Model file for the job. Use its own axes, mm. Face numbers are marked on the shaded views. A direction names the side the tool comes from. Coordinates: 2 decimals unless noted, no trailing zeros. Order: outer loops, then holes, each group sorted by start corner. A loop starts at its lowest first (then second) coordinate and runs counter-clockwise, first axis right, second up. Notation, with made-up numbers: (24, 43.25) -> (71, 43.25) arc R22 cw to (71, 59.25) -> close; hole circle Ø1 at (-1.5, 56.5). An arc over 180 degrees is marked (long way). Return JSON: item names as keys, results as strings. Group by question number.
1) Cut at B-B (y = 7.5). Write the cut outline in (x, z).
2) Which spindle directions (+Z, -Z, +X, -X, +Y, -Y) get a long thin tool onto all of the face, cutting with end or side? Do the marked faces 1, 2 and 3. Say none if no direction does.
3) Flat gauge pins, fed straight in: pin 1 (3 mm diameter, centred on x = -32, y = 3.5, fed in from +Z); pin 2 (2 mm diameter, centred on y = -9.5, z = 4, fed in from +X); pin 3 (20.5 mm diameter, centred on x = 17.5, y = 1, fed in from +Z). Where does each tip first touch, or does it go through?
4) Probe line 1 (Y direction, x = 0, z = 4); line 2 (X direction, y = -17, z = 11.5); line 3 (X direction, y = -4.5, z = 9.5). List the from-to ranges inside material, lowest first.
5) Pull direction X, two halves, no side cores. Call the marked faces 4, 5, 6 and 7: +X half, -X half, draft (parallel to the pull), parting line (faces both ways), or undercut.
6) Cut at C-C (y = 0). Write the cut outline in (x, z), and give its area (3 significant figures).
7) Cut at A-A (x = 0). Write the cut outline in (y, z), and give its area (3 significant figures).
8) Cut at D-D (x = 11). Write the cut outline in (y, z), and give its area (3 significant figures).
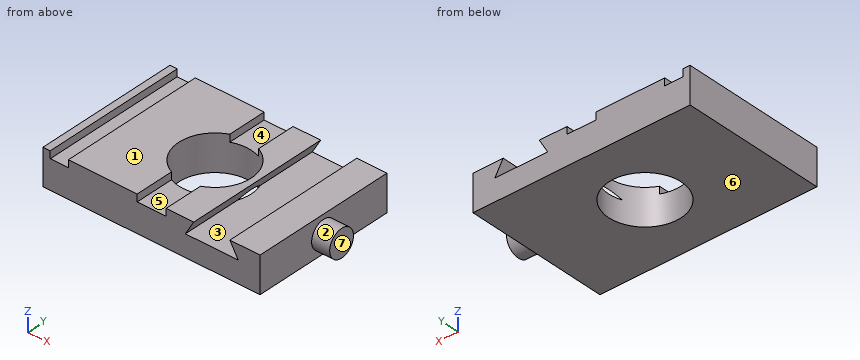
from build123d import *

# Parameters (mm, degrees)
F0_W     = 76.2
F0_H     = 50.8
F0_R     = 12.7
F1_DEPTH = 12.7
F2_W     = 6.35
F2_H     = 50.8
F3_DEPTH = 2.54
F5_DEPTH = 50.8
F6_R     = 4.7625
F7_DEPTH = 6.35


with BuildPart() as f1:
    # F0 (on Top) → F1 (new body)
    with BuildSketch(Plane.XY):
        Rectangle(F0_W, F0_H)
        Circle(F0_R, mode=Mode.SUBTRACT)
    extrude(amount=F1_DEPTH)

    # F2 (on face) → F3 (cut)
    with BuildSketch(Plane.XY.offset(12.7)):
        with Locations((-32.385, 0)):
            Rectangle(F2_W, F2_H)
        with BuildLine():
            Line((-5.039626, -11.65728), (-5.039626, -25.4))
            Line((-5.039626, -25.4), (5.120374, -25.4))
            Line((5.120374, -25.4), (5.120374, -11.622038))
            ThreePointArc((5.120374, -11.622038), (0.044052, -12.699924), (-5.039626, -11.65728))
        make_face()
        with BuildLine():
            Line((5.120374, 25.4), (-5.039626, 25.4))
            Line((-5.039626, 25.4), (-5.039626, 11.65728))
            ThreePointArc((-5.039626, 11.65728), (0.044052, 12.699924), (5.120374, 11.622038))
            Line((5.120374, 11.622038), (5.120374, 25.4))
        make_face()
    extrude(amount=-F3_DEPTH, mode=Mode.SUBTRACT)

    # F4 (on face) → F5 (cut, through all)
    with BuildSketch(Plane.XZ.offset(25.4)):
        Polygon((27.512688, 12.7), (14.812688, 12.7), (11.879749, 7.62), (30.445627, 7.62), align=None)
    extrude(amount=-F5_DEPTH, mode=Mode.SUBTRACT)

    # F6 (on face) → F7 (join)
    with BuildSketch(Plane.YZ.offset(38.1)):
        with Locations((0, 6.243965)):
            Circle(F6_R)
    extrude(amount=F7_DEPTH)


solid = f1.part
Answers below:
{
 "1": {"outline": "(-38.1, 0) -> (-10.25, 0) -> (-10.25, 12.7) -> (-29.21, 12.7) -> (-29.21, 10.16) -> (-35.56, 10.16) -> (-35.56, 12.7) -> (-38.1, 12.7) -> close; (10.25, 0) -> (38.1, 0) -> (38.1, 12.7) -> (27.51, 12.7) -> (30.45, 7.62) -> (11.88, 7.62) -> (14.81, 12.7) -> (10.25, 12.7) -> close"},
 "2": {"face 1": "+Z, +X, -X, +Y, -Y", "face 2": "+X", "face 3": "+Y, -Y"},
 "3": {"pin 1": "stops at z = 10.16", "pin 2": "stops at x = 38.1", "pin 3": "stops at z = 12.7"},
 "4": {"line 1": "y = -25.4 to -12.7, 12.7 to 25.4", "line 2": "x = -38.1 to -35.56, -29.21 to -5.04, 5.12 to 14.12, 28.21 to 38.1", "line 3": "x = -38.1 to -11.88, 11.88 to 12.97, 29.36 to 38.1"},
 "5": {"face 4": "undercut", "face 5": "undercut", "face 6": "draft", "face 7": "+X half"},
 "6": {"outline": "(-38.1, 0) -> (-12.7, 0) -> (-12.7, 12.7) -> (-29.21, 12.7) -> (-29.21, 10.16) -> (-35.56, 10.16) -> (-35.56, 12.7) -> (-38.1, 12.7) -> close; (12.7, 0) -> (38.1, 0) -> (38.1, 1.48) -> (44.45, 1.48) -> (44.45, 11.01) -> (38.1, 11.01) -> (38.1, 12.7) -> (27.51, 12.7) -> (30.45, 7.62) -> (12.7, 7.62) -> close; (12.7, 9.04) -> (14.81, 12.7) -> (12.7, 12.7) -> close", "area": "611 mm^2"},
 "7": {"outline": "(-25.4, 0) -> (-12.7, 0) -> (-12.7, 10.16) -> (-25.4, 10.16) -> close; (12.7, 0) -> (25.4, 0) -> (25.4, 10.16) -> (12.7, 10.16) -> close", "area": "258 mm^2"},
 "8": {"outline": "(-25.4, 0) -> (-6.35, 0) -> (-6.35, 12.7) -> (-25.4, 12.7) -> close; (6.35, 0) -> (25.4, 0) -> (25.4, 12.7) -> (6.35, 12.7) -> close", "area": "484 mm^2"}
}
